CAD build for the part. Positions are in the model's coordinates, mm. A direction names the side the tool comes from. Give positions to 0.01 mm unless a question says otherwise; leave off trailing zeros. Loops run counter-clockwise (first coordinate to the right, second up) from the corner with the lowest first, then second, coordinate; pieces in that order, holes last. Notation, with made-up numbers: (-4.5, 37) -> (21.5, 37) arc R27 cw to (21.5, 64) -> close; hole circle Ø8 at (-26.75, 88.25). An arc over 180 degrees is marked (long way). Use one line per item in the form item = value.
```python
from build123d import *

# Parameters (mm, degrees)
SKETCH1_W           = 122.28
SKETCH1_H           = 40
BOSS_EXTRUDE1_DEPTH = 10
SKETCH2_R           = 3.05
SKETCH2_R_2         = 1.25
CUT_EXTRUDE1_DEPTH  = 10
SKETCH3_R           = 1.25
CUT_EXTRUDE2_DEPTH  = 10
SKETCH4_R           = 5
BOSS_EXTRUDE2_DEPTH = 55
SKETCH5_R           = 14
BOSS_EXTRUDE3_DEPTH = 7.75
SKETCH10_W          = 7.75
SKETCH10_H          = 111.1
BOSS_EXTRUDE4_DEPTH = 28
SKETCH8_R           = 1.25
CUT_EXTRUDE6_DEPTH  = 7.75
CIRPATTERN2_COUNT   = 8
SKETCH6_R           = 5.05
CUT_EXTRUDE7_DEPTH  = 2
SKETCH11_R          = 2.675
CUT_EXTRUDE8_DEPTH  = 3
SKETCH14_W          = 30
SKETCH14_H          = 28
CUT_EXTRUDE10_DEPTH = 2.8
SKETCH15_R          = 1.25
CUT_EXTRUDE11_DEPTH = 10
SKETCH16_W          = 5.4
SKETCH16_H          = 8.6
SKETCH16_H_2        = 3.6
CUT_EXTRUDE12_DEPTH = 10
FILLET1_R           = 0.5
FILLET2_R           = 0.5
SKETCH17_W          = 54.68
SKETCH17_H          = 40
CUT_EXTRUDE14_DEPTH = 5
SKETCH18_W          = 26.65
SKETCH18_H          = 40
CUT_EXTRUDE15_DEPTH = 5
FILLET4_R           = 1.25
CUT_EXTRUDE17_REACH = 64.75
SKETCH21_W          = 15
SKETCH21_H          = 18
FILLET5_R           = 1.25
CUT_EXTRUDE18_REACH = 137.1
SKETCH22_W          = 14.65
SKETCH22_H          = 30
FILLET6_R           = 1.25
CUT_EXTRUDE19_REACH = 7
SKETCH23_W          = 12.14
SKETCH23_H          = 30
FILLET7_R           = 1.25


with BuildPart() as part:
    # Sketch1 → Boss-Extrude1 (new body)
    with BuildSketch(Plane.XY):
        with Locations((61.14, 20)):
            Rectangle(SKETCH1_W, SKETCH1_H)
    extrude(amount=BOSS_EXTRUDE1_DEPTH)

    # Sketch2 → Cut-Extrude1 (cut)
    with BuildSketch(Plane.XY.offset(10)):
        with Locations((61.14, 20)):
            Circle(SKETCH2_R)
        with Locations((76.14, 32.5)):
            Circle(SKETCH2_R_2)
        with Locations((76.14, 15.5)):
            Circle(SKETCH2_R_2)
    cut_extrude1 = extrude(amount=-CUT_EXTRUDE1_DEPTH, mode=Mode.SUBTRACT)

    # Mirror1: Cut-Extrude1 across plane
    add(cut_extrude1.mirror(Plane.ZY.offset(-61.14)), mode=Mode.SUBTRACT)

    # Sketch3 → Cut-Extrude2 (cut)
    with BuildSketch(Plane.ZY):
        with Locations((5, 20)):
            Circle(SKETCH3_R)
        with Locations((5, 30)):
            Circle(SKETCH3_R)
        with Locations((5, 10)):
            Circle(SKETCH3_R)
    cut_extrude2 = extrude(amount=-CUT_EXTRUDE2_DEPTH, mode=Mode.SUBTRACT)

    # Mirror2: Cut-Extrude2 across plane
    add(cut_extrude2.mirror(Plane.ZY.offset(-61.14)), mode=Mode.SUBTRACT)



with BuildPart() as body_2:
    # Sketch4 → Boss-Extrude2 (new body)
    with BuildSketch(Plane(origin=(76.43, 0, 0), x_dir=(0, 0, -1), z_dir=(1, 0, 0))):
        with Locations((-121.1, 20)):
            Circle(SKETCH4_R)
    extrude(amount=BOSS_EXTRUDE2_DEPTH)

    # Sketch5 → Boss-Extrude3 (add)
    with BuildSketch(Plane.ZY.offset(-76.43)):
        with Locations((121.1, 20)):
            Circle(SKETCH5_R)
    extrude(amount=BOSS_EXTRUDE3_DEPTH)


with BuildPart() as part_1:
    add(part.part)

    add(body_2.part)  # Boss-Extrude4 merges body 2
    # Sketch10 → Boss-Extrude4 (add)
    with BuildSketch(Plane(origin=(0, 6, 0), x_dir=(-1, 0, 0), z_dir=(0, -1, 0))):
        with Locations((-72.555, -65.55)):
            Rectangle(SKETCH10_W, SKETCH10_H)
    extrude(amount=-BOSS_EXTRUDE4_DEPTH)

    # Sketch8 → Cut-Extrude6 (cut)
    with BuildSketch(Plane.ZY.offset(-68.68)):
        with Locations((121.1, 9)):
            Circle(SKETCH8_R)
    cut_extrude6 = extrude(amount=-CUT_EXTRUDE6_DEPTH, mode=Mode.SUBTRACT)

    # CirPattern2: Cut-Extrude6 ×8 about axis
    cirpattern2_axis = Axis((0, 20, 121.1), (1, 0, 0))
    for i in range(1, CIRPATTERN2_COUNT):
        add(cut_extrude6.rotate(cirpattern2_axis, i * 360 / CIRPATTERN2_COUNT), mode=Mode.SUBTRACT)

    # Sketch6 → Cut-Extrude7 (cut)
    with BuildSketch(Plane.ZY.offset(-68.68)):
        with Locations((121.1, 20)):
            Circle(SKETCH6_R)
    extrude(amount=-CUT_EXTRUDE7_DEPTH, mode=Mode.SUBTRACT)

    # Sketch11 → Cut-Extrude8 (cut)
    with BuildSketch(Plane.ZY.offset(-70.68)):
        with Locations((121.1, 20)):
            Circle(SKETCH11_R)
    extrude(amount=-CUT_EXTRUDE8_DEPTH, mode=Mode.SUBTRACT)

    # Sketch14 → Cut-Extrude10 (cut)
    with BuildSketch(Plane(origin=(76.43, 0, 0), x_dir=(0, 0, -1), z_dir=(1, 0, 0))):
        with Locations((-25, 20)):
            Rectangle(SKETCH14_W, SKETCH14_H)
    extrude(amount=-CUT_EXTRUDE10_DEPTH, mode=Mode.SUBTRACT)

    # Sketch15 → Cut-Extrude11 (cut)
    with BuildSketch(Plane(origin=(0, 0, 0), x_dir=(-1, 0, 0), z_dir=(0, 0, -1))):
        with Locations((-86.14, 16)):
            Circle(SKETCH15_R)
        with Locations((-86.14, 36)):
            Circle(SKETCH15_R)
    cut_extrude11 = extrude(amount=-CUT_EXTRUDE11_DEPTH, mode=Mode.SUBTRACT)

    # Mirror3: Cut-Extrude11 across plane
    add(cut_extrude11.mirror(Plane.ZY.offset(-61.14)), mode=Mode.SUBTRACT)

    # Sketch16 → Cut-Extrude12 (cut)
    with BuildSketch(Plane(origin=(0, 0, 0), x_dir=(-1, 0, 0), z_dir=(0, 0, -1))):
        with Locations((-77.34, 35.3)):
            Rectangle(SKETCH16_W, SKETCH16_H)
        with Locations((-77.34, 15.8)):
            Rectangle(SKETCH16_W, SKETCH16_H_2)
    cut_extrude12 = extrude(amount=-CUT_EXTRUDE12_DEPTH, mode=Mode.SUBTRACT)

    # Mirror4: Cut-Extrude12 across plane
    add(cut_extrude12.mirror(Plane.ZY.offset(-61.14)), mode=Mode.SUBTRACT)

    # Fillet1
    fillet1_edges = [part_1.edges().sort_by_distance(p)[0] for p in [
        (74.64, 17.6, 5),
        (74.64, 14, 5),
        (80.04, 14, 5),
        (80.04, 17.6, 5),
        (47.64, 14, 5),
        (47.64, 17.6, 5),
        (42.24, 17.6, 5),
        (42.24, 14, 5),
    ]]
    fillet(fillet1_edges, radius=FILLET1_R)

    # Fillet2
    fillet2_edges = [part_1.edges().sort_by_distance(p)[0] for p in [
        (74.64, 39.6, 5),
        (74.64, 31, 5),
        (80.04, 31, 5),
        (80.04, 39.6, 5),
        (47.64, 31, 5),
        (47.64, 39.6, 5),
        (42.24, 39.6, 5),
        (42.24, 31, 5),
    ]]
    fillet(fillet2_edges, radius=FILLET2_R)

    # Sketch17 → Cut-Extrude14 (cut)
    with BuildSketch(Plane.XY.offset(10)):
        with Locations((39.34, 20)):
            Rectangle(SKETCH17_W, SKETCH17_H)
    extrude(amount=-CUT_EXTRUDE14_DEPTH, mode=Mode.SUBTRACT)

    # Sketch18 → Cut-Extrude15 (cut)
    with BuildSketch(Plane.XY.offset(10)):
        with Locations((96.955, 20)):
            Rectangle(SKETCH18_W, SKETCH18_H)
    extrude(amount=-CUT_EXTRUDE15_DEPTH, mode=Mode.SUBTRACT)

    # Fillet4
    fillet4_edges = [part_1.edges().sort_by_distance(p)[0] for p in [
        (66.68, 20, 10),
        (12, 20, 10),
        (110.28, 20, 10),
        (83.63, 20, 10),
    ]]
    fillet(fillet4_edges, radius=FILLET4_R)

    # Sketch21 → Cut-Extrude17 (cut, up to next)
    with BuildSketch(Plane.ZY.offset(-68.68), mode=Mode.PRIVATE) as cut_extrude17_sk1:
        with Locations((88.6, 20)):
            Rectangle(SKETCH21_W, SKETCH21_H)
    cut_extrude17_tool1 = extrude(cut_extrude17_sk1.sketch, amount=-CUT_EXTRUDE17_REACH, mode=Mode.PRIVATE) & part_1.part
    add(cut_extrude17_tool1.solids().sort_by_distance((68.68, 20, 88.6))[0], mode=Mode.SUBTRACT)
    # Sketch21 → Cut-Extrude17 (cut, up to next)
    with BuildSketch(Plane.ZY.offset(-68.68), mode=Mode.PRIVATE) as cut_extrude17_sk2:
        with Locations((68.6, 20)):
            Rectangle(SKETCH21_W, SKETCH21_H)
    cut_extrude17_tool2 = extrude(cut_extrude17_sk2.sketch, amount=-CUT_EXTRUDE17_REACH, mode=Mode.PRIVATE) & part_1.part
    add(cut_extrude17_tool2.solids().sort_by_distance((68.68, 20, 68.6))[0], mode=Mode.SUBTRACT)
    # Sketch21 → Cut-Extrude17 (cut, up to next)
    with BuildSketch(Plane.ZY.offset(-68.68), mode=Mode.PRIVATE) as cut_extrude17_sk3:
        with Locations((48.6, 20)):
            Rectangle(SKETCH21_W, SKETCH21_H)
    cut_extrude17_tool3 = extrude(cut_extrude17_sk3.sketch, amount=-CUT_EXTRUDE17_REACH, mode=Mode.PRIVATE) & part_1.part
    add(cut_extrude17_tool3.solids().sort_by_distance((68.68, 20, 48.6))[0], mode=Mode.SUBTRACT)
    # Sketch21 → Cut-Extrude17 (cut, up to next)
    with BuildSketch(Plane.ZY.offset(-68.68), mode=Mode.PRIVATE) as cut_extrude17_sk4:
        with Locations((28.6, 20)):
            Rectangle(SKETCH21_W, SKETCH21_H)
    cut_extrude17_tool4 = extrude(cut_extrude17_sk4.sketch, amount=-CUT_EXTRUDE17_REACH, mode=Mode.PRIVATE) & part_1.part
    add(cut_extrude17_tool4.solids().sort_by_distance((68.68, 20, 28.6))[0], mode=Mode.SUBTRACT)

    # Fillet5
    fillet5_edges = [part_1.edges().sort_by_distance(p)[0] for p in [
        (72.555, 29, 96.1),
        (72.555, 11, 96.1),
        (72.555, 11, 81.1),
        (72.555, 29, 81.1),
        (72.555, 29, 76.1),
        (72.555, 11, 76.1),
        (72.555, 11, 61.1),
        (72.555, 29, 61.1),
        (72.555, 29, 56.1),
        (72.555, 11, 56.1),
        (72.555, 11, 41.1),
        (72.555, 29, 41.1),
        (71.155, 29, 36.1),
        (71.155, 11, 36.1),
        (71.155, 11, 21.1),
        (71.155, 29, 21.1),
    ]]
    fillet(fillet5_edges, radius=FILLET5_R)

    # Sketch22 → Cut-Extrude18 (cut, up to next)
    with BuildSketch(Plane(origin=(0, 0, 0), x_dir=(-1, 0, 0), z_dir=(0, 0, -1)), mode=Mode.PRIVATE) as cut_extrude18_sk1:
        with Locations((-96.955, 20)):
            Rectangle(SKETCH22_W, SKETCH22_H)
    cut_extrude18_tool1 = extrude(cut_extrude18_sk1.sketch, amount=-CUT_EXTRUDE18_REACH, mode=Mode.PRIVATE) & part_1.part
    add(cut_extrude18_tool1.solids().sort_by_distance((96.955, 20, 0))[0], mode=Mode.SUBTRACT)

    # Fillet6
    fillet6_edges = [part_1.edges().sort_by_distance(p)[0] for p in [
        (89.63, 5, 2.5),
        (89.63, 35, 2.5),
        (104.28, 35, 2.5),
        (104.28, 5, 2.5),
    ]]
    fillet(fillet6_edges, radius=FILLET6_R)

    # Sketch23 → Cut-Extrude19 (cut, up to next)
    with BuildSketch(Plane.XY.offset(5), mode=Mode.PRIVATE) as cut_extrude19_sk1:
        with Locations((24.07, 20)):
            Rectangle(SKETCH23_W, SKETCH23_H)
    cut_extrude19_tool1 = extrude(cut_extrude19_sk1.sketch, amount=-CUT_EXTRUDE19_REACH, mode=Mode.PRIVATE) & part_1.part
    add(cut_extrude19_tool1.solids().sort_by_distance((24.07, 20, 5))[0], mode=Mode.SUBTRACT)

    # Fillet7
    fillet7_edges = [part_1.edges().sort_by_distance(p)[0] for p in [
        (18, 5, 2.5),
        (18, 35, 2.5),
        (30.14, 35, 2.5),
        (30.14, 5, 2.5),
    ]]
    fillet(fillet7_edges, radius=FILLET7_R)


solid = part_1.part
```
1. Tool access for faces 1 (the flat face through (80.04, 35, 5)), 2 (the flat face through (70.68, 17.8, 123.3)), 3 (the flat face through (73, 20, 81.1)), 4 (the flat face through (74.64, 35, 5)): list every direction of +Z, -Z, +X, -X, +Y, -Y with a clear straight run to the whole face (end or side of a thin tool).
Result sheet:
face_1 = +Z, -Z
face_2 = -X
face_3 = +X, -X
face_4 = -Z
2. Mould opens along X. For faces 5 (the flat face through (68.68, 30, 72)), 6 (the flat face through (18, 20, 3)), 7 (the flat face through (76.43, 20, 97)), 8 (the flat face through (77, 31, 5)) say: pulls with the +X half, pulls with the -X half, needs draft (parallel to the pull), parting line crosses it, or undercut.
Result sheet:
face_5 = pulls with the -X half
face_6 = undercut
face_7 = pulls with the +X half
face_8 = undercut
3. Drill centre lines: line 1 (Y direction, x = 86.14, z = 2.65); line 2 (Y direction, x = 116.25, z = 5); line 3 (X direction, y = 7.5, z = 59.5). Where is each one in solid material? Low to high.
Result sheet:
line_1 = 0 to 14.75, 17.25 to 34.75, 37.25 to 40
line_2 = 0 to 8.75, 11.25 to 18.75, 21.25 to 28.75, 31.25 to 40
line_3 = 68.68 to 76.43
4. Drop flat-ended pins along their axis: P1, Ø2, axis at y = 30.5, z = 41.5, coming from the -X side; P2, Ø5, axis at x = 109.5, y = 18, coming from the -Z side; P3, Ø4, axis at x = 73.5, z = 50.5, coming from the +Y side; P4, Ø1.5, axis at y = 20, z = 5, coming from the +X side. Give the stop position or say it passes through.
Result sheet:
P1 = 68.68
P2 = 0
P3 = 34
P4 = 112.28
5. Cut at A-A, the plane x = 45. Write the cut outline in (y, z), then the cut area to 3 significant figures.
Result sheet:
outline = (0, 0) -> (14, 0) -> (14, 5) -> (0, 5) -> close; (17.6, 0) -> (31, 0) -> (31, 5) -> (17.6, 5) -> close; (39.6, 0) -> (40, 0) -> (40, 5) -> (39.6, 5) -> close
area = 139 mm^2
